Design review of the part built by this model. Coordinates are the model's own, in mm. A direction names the side the tool comes from. Coordinates: 2 decimals unless noted, no trailing zeros. Write each loop counter-clockwise with the first axis right and the second up, starting at its lowest first coordinate (ties: lowest second). Pieces come first, ordered by that corner, then holes.
Q1. Take a section at A-A (y = 5.25). Give the boundary of the cut face in (x, z).
Q2. Take a section at C-C (y = -0.75). Give the boundary of the cut face in (x, z).
Q3. Take a section at D-D (z = 2). Give the boundary of the cut face in (x, y), and give its area (3 significant figures).
Q4. Insertion check: pin 1 (2.5 mm diameter, centred on x = 0.5, z = 0, fed in from +Y); pin 2 (1.5 mm diameter, centred on y = -1.5, z = -0.5, fed in from +X); pin 3 (0.9 mm diameter, centred on x = 0, y = -2, fed in from +Z). Each pin has a flat end and moves straight along its axis. Give the tip position at first contact, or say it passes through.
Q5. Mouldability with a two-part tool opening along X and no side actions: class faces 1 (the flat face through (2.5, -1, 0)), 2 (the flat face through (0, 8, -2)), 3 (the flat face through (-2.5, 6, 0)) as pulls with the +X half, pulls with the -X half, needs draft (parallel to the pull), parting line crosses it, or undercut.
Q6. For probe 1 along X at (y, z) = (5, 0.5); probe 2 along Z at (x, y) = (1.5, 6.25); probe 3 along Y at (x, z) = (-3.5, -5.5), list the stretches that pass through material, from the lowest coordinate up.
Q7. Machinability: for faces 4 (the flat face through (0, 6, 1.5)), 5 (the flat face through (-2.5, -1, 0)), 6 (the flat face through (0, -1, 1.5)), which of the approach directions +Z, -Z, +X, -X, +Y, -Y give a long, thin tool a straight path to every point of the face, cutting with its end or side? Answer none if there is none.
Q8. Take a section at B-B (x = 0.75). Give the boundary of the cut face in (y, z).
```python
from build123d import *

# Parameters (mm, degrees)
SKETCH1_W           = 20
SKETCH1_H           = 15
BOSS_EXTRUDE1_DEPTH = 8
SKETCH2_W           = 5
SKETCH2_H           = 3
CUT_EXTRUDE1_DEPTH  = 3.2
SKETCH3_W           = 5
SKETCH3_H           = 3
BOSS_EXTRUDE2_DEPTH = 3


with BuildPart() as part:
    # Sketch1 → Boss-Extrude1 (new body)
    with BuildSketch(Plane(origin=(0, 0, 0), x_dir=(1, 0, 0), z_dir=(0, 1, 0))):
        Rectangle(SKETCH1_W, SKETCH1_H)
    extrude(amount=BOSS_EXTRUDE1_DEPTH)

    # Sketch2 → Cut-Extrude1 (cut)
    with BuildSketch(Plane(origin=(0, 8, 0), x_dir=(1, 0, 0), z_dir=(0, 1, 0))):
        Rectangle(SKETCH2_W, SKETCH2_H)
    extrude(amount=-CUT_EXTRUDE1_DEPTH, mode=Mode.SUBTRACT)

    # Sketch3 → Boss-Extrude2 (add)
    with BuildSketch(Plane.XZ):
        Rectangle(SKETCH3_W, SKETCH3_H)
    extrude(amount=BOSS_EXTRUDE2_DEPTH)


solid = part.part
```
Response:
1. outline: (-10, -7.5) - (10, -7.5) - (10, 7.5) - (-10, 7.5) - close; hole (-2.5, -1.5) - (2.5, -1.5) - (2.5, 1.5) - (-2.5, 1.5) - close
2. outline: (-2.5, -1.5) - (2.5, -1.5) - (2.5, 1.5) - (-2.5, 1.5) - close
3. outline: (-10, 0) - (10, 0) - (10, 8) - (-10, 8) - close
3. area: 160 mm2
4. pin 1: stops at y = 4.8
4. pin 2: stops at x = 2.5
4. pin 3: stops at z = 1.5
5. face 1: pulls with the +X half
5. face 2: needs draft
5. face 3: undercut
6. probe 1: x = -10 to -2.5, 2.5 to 10
6. probe 2: z = -7.5 to -1.5, 1.5 to 7.5
6. probe 3: y = 0 to 8
7. face 4: +Y
7. face 5: +Z, -Z, -X, -Y
7. face 6: +Z, +X, -X, -Y
8. outline: (-3, -1.5) - (0, -1.5) - (0, -7.5) - (8, -7.5) - (8, -1.5) - (4.8, -1.5) - (4.8, 1.5) - (8, 1.5) - (8, 7.5) - (0, 7.5) - (0, 1.5) - (-3, 1.5) - close
